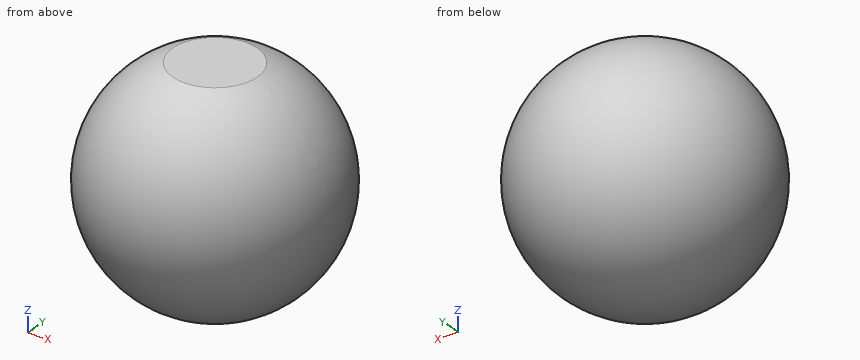
from build123d import *

# Parameters (mm, degrees)
F3_W     = 33.02
F3_H     = 33.02
F4_DEPTH = 25.4
F5_T     = -0.5


with BuildPart() as f1:
    # F0 (on Front) → F1 (revolve)
    with BuildSketch(Plane.XZ):
        with BuildLine():
            Line((0, 38.1), (0, -38.1))
            ThreePointArc((0, -38.1), (38.1, 0), (0, 38.1))
        make_face()
    revolve(axis=Axis((0, 0, 0), (0, 0, -1)))

    # F3 (on offset) → F4 (cut)
    with BuildSketch(Plane.XY.offset(35.56)):
        Rectangle(F3_W, F3_H)
    extrude(amount=F4_DEPTH, mode=Mode.SUBTRACT)

    # F5 (hollow: no face is removed)
    offset(amount=F5_T, mode=Mode.SUBTRACT)


solid = f1.part
Model file for the job. Use its own axes, mm. Round coordinates to 2 decimals unless told otherwise and drop trailing zeros. Loops run counter-clockwise (first coordinate to the right, second up) from the corner with the lowest first, then second, coordinate; pieces in that order, holes last. Notation, with made-up numbers: (-20, 2) - (13, 2) arc R7 ccw to (13, 6) - close; hole circle Ø5 at (46, 15.5). An arc over 180 degrees is marked (long way). Write each question's results on one line, items separated by ' | '.
(1) Saw through at C-C, the plane x = -12.5. List the corners of the cut face in (y, z).
Answer below:
outline: (-5.55, 35.56) arc R35.99 ccw (long way) to (5.55, 35.56) - close; hole (-5.32, 35.06) arc R35.46 ccw (long way) to (5.32, 35.06) - close
(2) Saw through at B-B, the plane y = -26. List the corners of the cut face in (x, z), then the cut area to 3 significant figures.
Answer below:
outline: circle Ø55.7 at (0, 0); hole circle Ø54.32 at (0, 0) | area: 119 mm^2
(3) Pin check, flat tips, straight feed: pin 1 (2 mm diameter, centred on x = -3.5, z = -26, fed in from +Y); pin 2 (4 mm diameter, centred on y = -20.5, z = -26, fed in from +X); pin 3 (10 mm diameter, centred on y = 19, z = -7, fed in from -X). Stop position of each tip, or through.
Answer below:
pin 1: stops at y = 28.55 | pin 2: stops at x = 22 | pin 3: stops at x = -34.92
(4) Saw through at D-D, the plane y = 9.5. List the corners of the cut face in (x, z), then the cut area to 3 significant figures.
Answer below:
outline: (-9.84, 35.56) arc R36.9 ccw (long way) to (9.84, 35.56) - close; hole (-9.71, 35.06) arc R36.38 ccw (long way) to (9.71, 35.06) - close | area: 118 mm^2
(5) Saw through at A-A, the plane z = 3.5. List the corners of the cut face in (x, y), then the cut area to 3 significant figures.
Answer below:
outline: circle Ø75.88 at (0, 0); hole circle Ø74.87 at (0, 0) | area: 119 mm^2
(6) Wall check: L1, parallel to Z at x = 16, y = 30.5; L2, parallel to X at y = 30, z = -2.5; L3, parallel to Z at x = 7, y = -22.5. Give the ranges that are in metal, low to high.
Answer below:
L1: z = -16.29 to -15.08, 15.08 to 16.29 | L2: x = -23.35 to -22.53, 22.53 to 23.35 | L3: z = -29.94 to -29.3, 29.3 to 29.94
